```python
from build123d import *

# Parameters (mm, degrees)
BOSS_EXTRUDE1_START = 2
SKETCH2_R           = 3
BOSS_EXTRUDE1_DEPTH = 2
CIRPATTERN1_COUNT   = 3
HOLE3_D             = 30
HOLE3_CBORE_D       = 46
HOLE3_CBORE_DEPTH   = 4
FILLET1_R           = 6
SKETCH9_R           = 30
SKETCH9_R_2         = 4
BOSS_EXTRUDE2_DEPTH = 5
HOLE4_D             = 6
HOLE4_DEPTH         = 5


with BuildPart() as part:
    # Sketch1 → Revolve1 (revolve)
    with BuildSketch(Plane.XY, mode=Mode.PRIVATE) as revolve1_sk:
        Polygon((0, 0), (0, 10), (17, 10), (17, 30), (12, 30), (12, 34), (42, 34), (42, 0), align=None)
    revolve(revolve1_sk.sketch.rotate(Axis((42, 34, 0), (0, -1, 0)), 270), axis=Axis((42, 34, 0), (0, -1, 0)))

    # Sketch2 → Boss-Extrude1 (add)
    with BuildSketch(Plane(origin=(0, 0, 0), x_dir=(1, 0, 0), z_dir=(0, 1, 0)).offset(BOSS_EXTRUDE1_START)):
        with BuildLine():
            Line((37, 55), (47, 55))
            ThreePointArc((47, 55), (50.535533906, 53.535533906), (52, 50))
            Line((52, 50), (52, 40.792156109))
            ThreePointArc((52, 40.792156109), (42, 42), (32, 40.792156109))
            Line((32, 40.792156109), (32, 50))
            ThreePointArc((32, 50), (33.464466094, 53.535533906), (37, 55))
        make_face()
        with Locations(Location((42, 48, 0), (0, 0, 270))):
            Circle(SKETCH2_R, mode=Mode.SUBTRACT)
    boss_extrude1 = extrude(amount=-BOSS_EXTRUDE1_DEPTH)

    # CirPattern1: Boss-Extrude1 ×3 about axis
    cirpattern1_axis = Axis((42, 0, 0), (0, 1, 0))
    for i in range(1, CIRPATTERN1_COUNT):
        add(boss_extrude1.rotate(cirpattern1_axis, i * 360 / CIRPATTERN1_COUNT))

    # Hole3 (through all)
    with Locations(Plane(origin=(0, 34, 0), x_dir=(1, 0, 0), z_dir=(0, 1, 0))):
        with Locations((42, 0)):
            CounterBoreHole(HOLE3_D / 2, HOLE3_CBORE_D / 2, HOLE3_CBORE_DEPTH)

    # Fillet1
    fillet1_edges = [part.edges().sort_by_distance(p)[0] for p in [
        (57, 30, 0),
        (42, 10, -42),
    ]]
    fillet(fillet1_edges, radius=FILLET1_R)

    # Sketch9 → Boss-Extrude2 (add)
    with BuildSketch(Plane(origin=(0, 34, 0), x_dir=(1, 0, 0), z_dir=(0, 1, 0))):
        with BuildLine():
            Line((84.405889748, 35), (84.405889748, 23))
            Line((84.405889748, 23), (87, 23))
            Line((87, 23), (87, 8))
            Line((87, 8), (83.231056256, 8))
            ThreePointArc((83.231056256, 8), (83.908844823, -2.76563295), (81.822211706, -13.348837209))
            ThreePointArc((81.822211706, -13.348837209), (80.749412141, -22.553158791), (83.47715359, -31.409222322))
            ThreePointArc((83.47715359, -31.409222322), (82.131599646, -40.339839701), (73.15454759, -41.329273159))
            ThreePointArc((73.15454759, -41.329273159), (42, -32.606891712), (10.84545241, -41.329273159))
            ThreePointArc((10.84545241, -41.329273159), (1.868400354, -40.339839701), (0.52284641, -31.409222322))
            ThreePointArc((0.52284641, -31.409222322), (3.250587859, -22.553158791), (2.177788294, -13.348837209))
            ThreePointArc((2.177788294, -13.348837209), (0.091155177, -2.76563295), (0.768943744, 8))
            Line((0.768943744, 8), (-3, 8))
            Line((-3, 8), (-3, 23))
            Line((-3, 23), (-0.405889748, 23))
            Line((-0.405889748, 23), (-0.405889748, 35))
            ThreePointArc((-0.405889748, 35), (3.369007961, 41.454695947), (10.84545241, 41.329273159))
            ThreePointArc((10.84545241, 41.329273159), (42, 32.606891712), (73.15454759, 41.329273159))
            ThreePointArc((73.15454759, 41.329273159), (80.630992039, 41.454695947), (84.405889748, 35))
        make_face()
        with Locations(Location((42, 0, 0), (0, 0, 270))):
            Circle(SKETCH9_R, mode=Mode.SUBTRACT)
        with Locations(Location((77, 35, 0), (0, 0, 270))):
            Circle(SKETCH9_R_2, mode=Mode.SUBTRACT)
        with Locations(Location((77, -35, 0), (0, 0, 270))):
            Circle(SKETCH9_R_2, mode=Mode.SUBTRACT)
        with Locations(Location((7, -35, 0), (0, 0, 270))):
            Circle(SKETCH9_R_2, mode=Mode.SUBTRACT)
        with Locations(Location((7, 35, 0), (0, 0, 270))):
            Circle(SKETCH9_R_2, mode=Mode.SUBTRACT)
    extrude(amount=-BOSS_EXTRUDE2_DEPTH)

    # Hole4
    with Locations(Plane(origin=(0, 34, 0), x_dir=(1, 0, 0), z_dir=(0, 1, 0))):
        with Locations((9, 16.4)):
            Hole(HOLE4_D / 2, depth=HOLE4_DEPTH)


solid = part.part
```
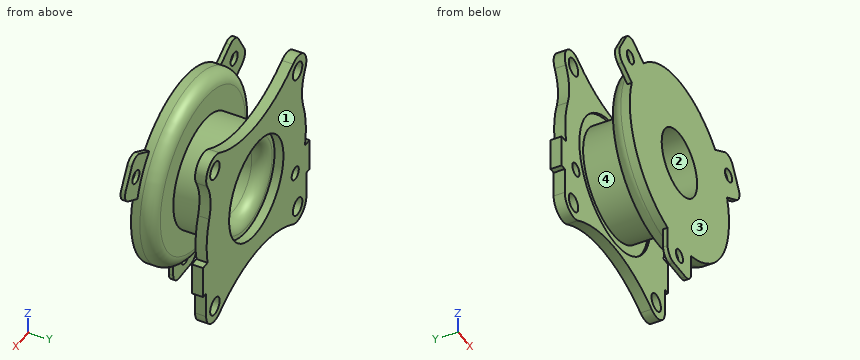
Model file for the job. Use its own axes, mm. Face numbers are marked on the shaded views. A direction names the side the tool comes from. Coordinates: 2 decimals unless noted, no trailing zeros. Order: outer loops, then holes, each group sorted by start corner. A loop starts at its lowest first (then second) coordinate and runs counter-clockwise, first axis right, second up. Notation, with made-up numbers: (36, 61.5) - (63, 61.5) arc R20 cw to (63, 93.5) - close; hole circle Ø7 at (33, -4). An arc over 180 degrees is marked (long way). Return JSON: item names as keys, results as strings. Group by question number.
1) Tool access for the marked faces 3 and 4: list every direction of +Z, -Z, +X, -X, +Y, -Y with a clear straight run to the whole face (end or side of a thin tool).
2) Saw through at A-A, the plane y = 22.5. Write the cut outline in (x, z), plus the area to 3 significant figures.
3) Saw through at C-C, the plane y = 5.5. Write the cut outline in (x, z).
4) Mould opens along Z. For the marked faces 1 and 2 say: released by +Z, released by -Z, zero draft, split by the parting line, or undercut.
5) Flat gauge pins, fed straight in: P1, Ø2, axis at y = 6.5, z = -11, coming from the +X side; P2, Ø1.5, axis at y = 32, z = -15.5, coming from the -X side; P3, Ø2, axis at x = 85.5, y = 32.5, coming from the -Z side. Where does each tip first touch, or does it go through?
6) Probe line 1 (Y direction, x = 68.5, z = -0.5); line 2 (Y direction, x = 79.5, z = 22); line 3 (Z direction, x = 37, y = 16.5). List the from-to ranges inside material, lowest first. Write a range as from..to.
7) Saw through at B-B, the plane x = 9. Count the separate pieces of the cut face and the enclosed holes in it, plus the area to 3 significant figures.
Values found:
{
 "1": {"face 3": "+Z, -Z, +X, -X, -Y", "face 4": "none"},
 "2": {"outline": "circle Ø50 at (42, 0); hole circle Ø30 at (42, 0)", "area": "1,260 mm²"},
 "3": {"outline": "circle Ø83.62 at (42, 0); hole circle Ø30 at (42, 0)"},
 "4": {"face 1": "zero draft", "face 2": "undercut"},
 "5": {"P1": "stops at x = 82.44", "P2": "stops at x = -3", "P3": "stops at z = -23"},
 "6": {"line 1": "y = 0..10, 30..34", "line 2": "y = 0..2, 29..34", "line 3": "z = -24.49..-14.14, 14.14..24.49"},
 "7": {"separate pieces": "5", "enclosed holes": "0", "area": "824 mm²"}
}
